Geometry: see drawing. Coordinates: mm, zero at the bounding-box minimum. A direction names the side the tool comes from. Round coordinates to 2 decimals unless told otherwise and drop trailing zeros. Loops run counter-clockwise (first coordinate to the right, second up) from the corner with the lowest first, then second, coordinate; pieces in that order, holes last. Notation, with made-up numbers: (-19.5, 68) -> (-14.5, 68) arc R20 ccw to (-14.5, 84) -> close; hole circle Ø11 at (-0.75, 10.25). An arc over 180 degrees is marked (long way). Answer in a Markdown table with one row per item.
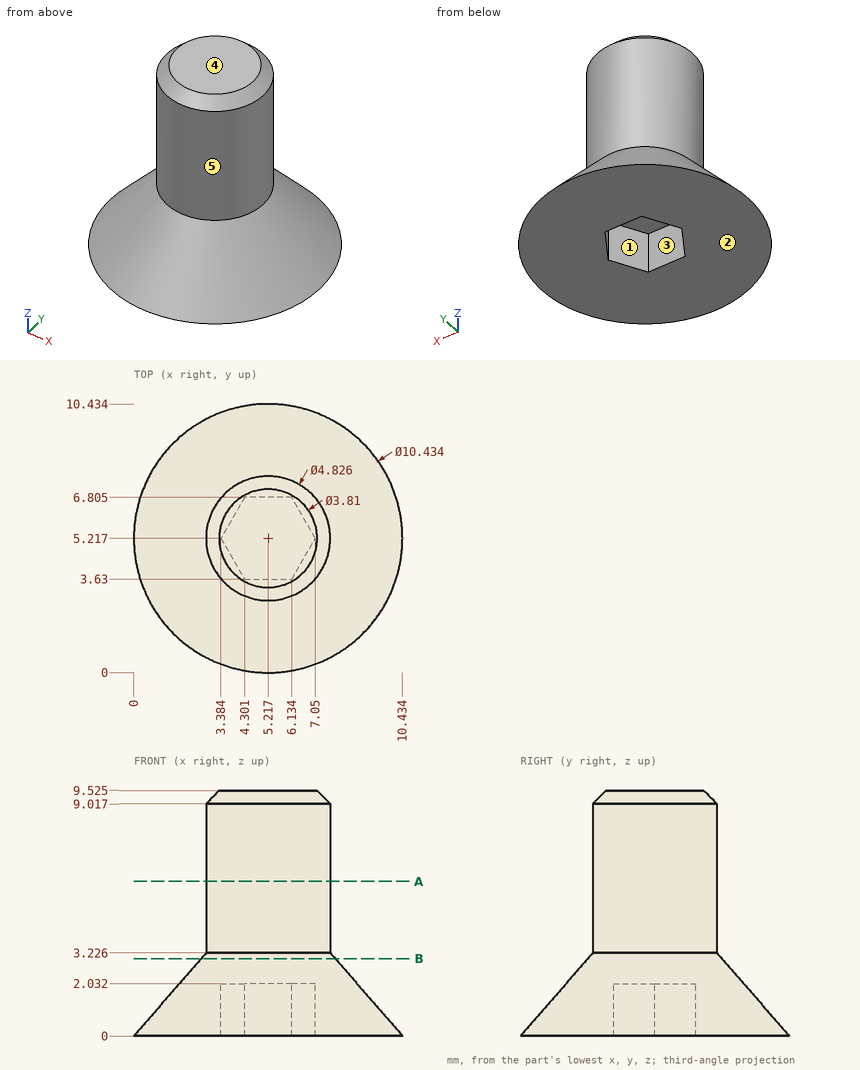
Item 1: Mould query, pull axis Y, two halves, no side actions, for the marked faces 3, 4 and 5. Classes: released by +Y, released by -Y, zero draft, split by the parting line, or undercut.
Ans:
| item | result |
|---|---|
| face 3 | undercut |
| face 4 | zero draft |
| face 5 | split by the parting line |
Item 2: First-contact query: P1, Ø1, axis at x = 5.5, z = 6.5, coming from the -Y side; P2, Ø1.5, axis at y = 3, z = 2, coming from the -X side; P3, Ø0.5, axis at x = 5, z = 0.5, coming from the -Y side. Flat tips, straight axial feed; report the tip coordinate or a pass-through.
Ans:
| item | result |
|---|---|
| P1 | y = 2.8 |
| P2 | x = 1.62 |
| P3 | y = 0.22 |
Item 3: Ray query, L1, parallel to X at y = 5, z = 1.25 (1 decimal); L2, parallel to Z at x = 4.5, y = 5.25 (1 decimal); L3, parallel to Y at x = 5.5, z = 1.75 (1 decimal). Return the intervals inside material, ascending.
Ans:
| item | result |
|---|---|
| L1 | 1.1 to 3.5, 6.9 to 9.3 |
| L2 | 2 to 9.5 |
| L3 | 1.5 to 3.6, 6.8 to 8.9 |
Item 4: Set-up query: the marked faces 1 and 2. Return all of +Z, -Z, +X, -X, +Y, -Y with unobstructed straight access to the full face (end or side cutting, diameter ignored); none if empty.
Ans:
| item | result |
|---|---|
| face 1 | -Z |
| face 2 | -Z, +X, -X, +Y, -Y |
Item 5: Section query B-B, the plane z = 3. Output: boundary loops of the cut face in (x, y).
Ans:
| item | result |
|---|---|
| outline | circle Ø5.22 at (5.22, 5.22) |
Item 6: Section query A-A, the plane z = 6. Output: boundary loops of the cut face in (x, y).
Ans:
| item | result |
|---|---|
| outline | circle Ø4.83 at (5.22, 5.22) |
